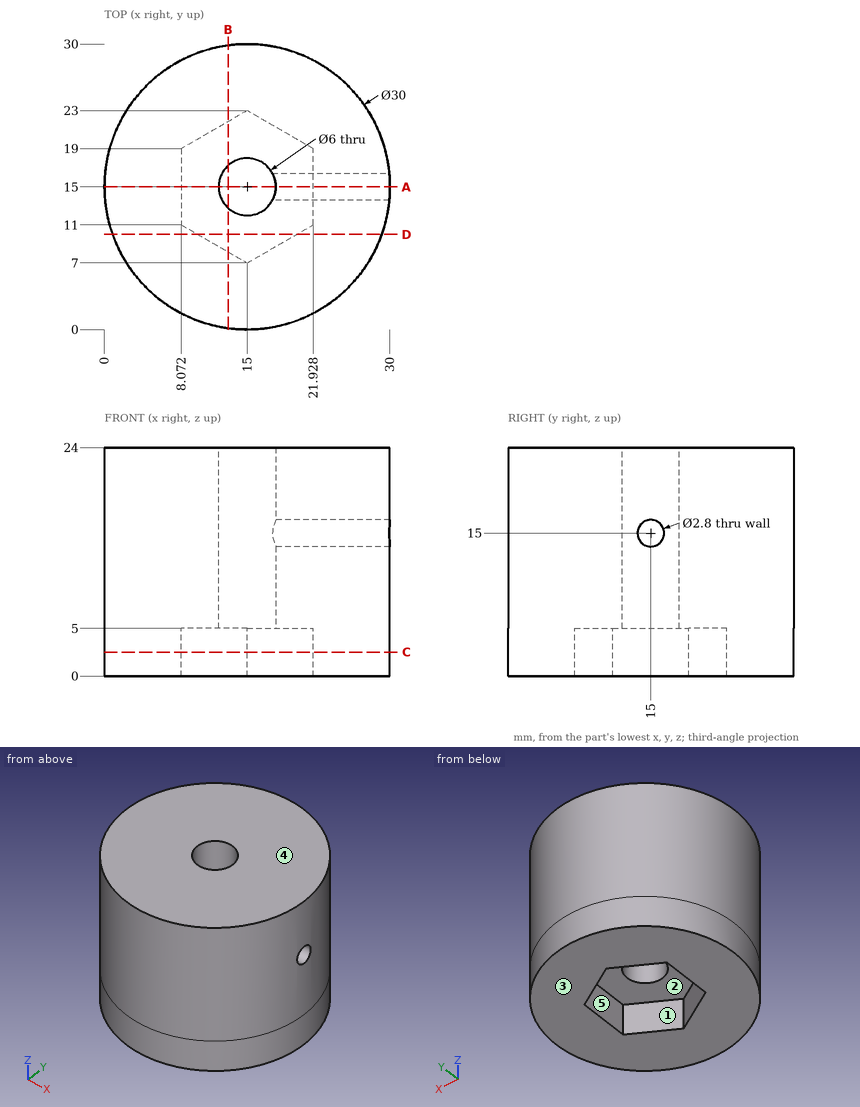
The drawing under review shows one solid part. Ordinate dimensions are in mm from its lowest x, y, z. A direction names the side the tool comes from. Coordinates: 2 decimals unless noted, no trailing zeros. Order: outer loops, then holes, each group sorted by start corner. A loop starts at its lowest first (then second) coordinate and runs counter-clockwise, first axis right, second up. Notation, with made-up numbers: (-14.5, 68) -> (13.5, 68) arc R26 ccw to (13.5, 104) -> close; hole circle Ø8 at (48.25, 88). An arc over 180 degrees is marked (long way). Use CSV: the item, a comma, the result in double quotes. Start each with the question number.
Item 1: We need section C-C, the plane z = 2.5. Give the boundary of the cut face in (x, y), then the cut area to 3 significant figures.
Item 2: We need section B-B, the plane x = 13. Give the boundary of the cut face in (y, z) (1 decimal), then the cut area to 3 significant figures.
Item 3: Draft analysis for pull direction Y (two halves, no side actions). For the marked faces 1, 2 and 3, state which applies: pulls with the +Y half, pulls with the -Y half, needs draft (parallel to the pull), parting line crosses it, or undercut.
Item 4: We need section A-A, the plane y = 15. Give the boundary of the cut face in (x, z).
Item 5: For the marked faces 4 and 5, list the 3-axis set-ups (+Z, -Z, +X, -X, +Y, -Y) from which the entire face can be reached by the end or side of a thin tool; tool diameter is ignored.
Item 6: Insertion check: pin 1 (1.5 mm diameter, centred on x = 11.5, z = 6.5, fed in from +Y); pin 2 (7 mm diameter, centred on x = 17.5, y = 13.5, fed in from -Z); pin 3 (5 mm diameter, centred on y = 22.5, z = 16, fed in from -X). Each pin has a flat end and moves straight along its axis. Give the tip position at first contact, or say it passes through.
Item 7: We need section D-D, the plane y = 10. Give the boundary of the cut face in (x, z), then the cut area to 3 significant figures.
Item 8: Wall thickness on probe 1 along Y at (x, z) = (15, 13); probe 2 along Z at (x, y) = (18.5, 11); probe 3 along X at (y, z) = (15.5, 11): over which ranges is each line inside the solid? List them lowest first.
Derived:
1,outline,"circle Ø30 at (15, 15); hole (8.07, 11) -> (15, 7) -> (21.93, 11) -> (21.93, 19) -> (15, 23) -> (8.07, 19) -> close"
1,area,"541 mm^2"
2,outline,"(0.1, 0) -> (8.2, 0) -> (8.2, 5) -> (12.8, 5) -> (12.8, 24) -> (0.1, 24) -> close; (17.2, 5) -> (21.8, 5) -> (21.8, 0) -> (29.9, 0) -> (29.9, 24) -> (17.2, 24) -> close"
2,area,"560 mm^2"
3,face 1,"undercut"
3,face 2,"undercut"
3,face 3,"needs draft"
4,outline,"(0, 0) -> (8.07, 0) -> (8.07, 5) -> (12, 5) -> (12, 24) -> (0, 24) -> close; (18, 5) -> (21.93, 5) -> (21.93, 0) -> (30, 0) -> (30, 13.6) -> (18, 13.6) -> close; (18, 16.4) -> (30, 16.4) -> (30, 24) -> (18, 24) -> close"
5,face 4,"+Z, +X, -X, +Y, -Y"
5,face 5,"-Z"
6,pin 1,"stops at y = 29.75"
6,pin 2,"stops at z = 5"
6,pin 3,"stops at x = 0.86"
7,outline,"(0.86, 0) -> (9.8, 0) -> (9.8, 5) -> (20.2, 5) -> (20.2, 0) -> (29.14, 0) -> (29.14, 24) -> (0.86, 24) -> close"
7,area,"627 mm^2"
8,probe 1,"y = 0 to 12, 18 to 30"
8,probe 2,"z = 5 to 24"
8,probe 3,"x = 0.01 to 12.04, 17.96 to 29.99"
